Read the model definition and answer for the solid it produces. Units are mm, in the model's axes. A direction names the side the tool comes from. Round coordinates to 2 decimals unless told otherwise and drop trailing zeros. Loops run counter-clockwise (first coordinate to the right, second up) from the corner with the lowest first, then second, coordinate; pieces in that order, holes last. Notation, with made-up numbers: (28.25, 71.5) -> (32.25, 71.5) arc R17 cw to (32.25, 77.5) -> close; hole circle Ø9 at (53.5, 66.5). An arc over 180 degrees is marked (long way). Put each result on its own line as item: value.
from build123d import *

# Parameters (mm, degrees)
F0_W         = 20
F0_H         = 20
F0_R         = 8.25
F1_DEPTH     = 28.5
F0_R_2       = 4.75
F2_DEPTH     = 1.5
F3_W         = 9
F3_H         = 17.5
F3_R         = 1.6
F4_DEPTH     = 10
F5_W         = 9
F5_H         = 17.5
F6_DEPTH     = 10
F7_DEPTH     = 30.001
F8_R         = 5
F9_T1_DEPTH  = 22.5
F10_T1_DEPTH = 22.5
F11_R        = 1


# Not quite as in the source:
# - a fillet or chamfer that OpenCascade refuses, or shapes differently, is made with other operations: its cross-section is extruded or revolved along the edge and cut away or added


with BuildPart() as f1:
    # F0 (on Top) → F1 (new body)
    with BuildSketch(Plane.XY):
        Rectangle(F0_W, F0_H)
        Circle(F0_R, mode=Mode.SUBTRACT)
    extrude(amount=F1_DEPTH)

    # F0 (on Top) → F2 (join)
    with BuildSketch(Plane.XY):
        Circle(F0_R)
        Circle(F0_R_2, mode=Mode.SUBTRACT)
    extrude(amount=F2_DEPTH)

    # F3 (on face) → F4 (join)
    with BuildSketch(Plane(origin=(-10, 0, 0), x_dir=(0, -1, 0), z_dir=(-1, 0, 0))):
        with Locations((0, 8.75)):
            Rectangle(F3_W, F3_H)
        with Locations((0, 8.75)):
            Circle(F3_R, mode=Mode.SUBTRACT)
    extrude(amount=F4_DEPTH)

    # F5 (on face) → F6 (join)
    with BuildSketch(Plane.YZ.offset(10)):
        with Locations((0, 8.75)):
            Rectangle(F5_W, F5_H)
    extrude(amount=F6_DEPTH)

    # F3 (on face) → F7 (cut, through all)
    with BuildSketch(Plane(origin=(-10, 0, 0), x_dir=(0, -1, 0), z_dir=(-1, 0, 0))):
        with Locations((0, 8.75)):
            Circle(F3_R)
    extrude(amount=-F7_DEPTH, mode=Mode.SUBTRACT)

    # F8
    f8_edges = [f1.edges().sort_by_distance(p)[0] for p in [
        (-10, -10, 14.25),
        (10, -10, 14.25),
        (10, 10, 14.25),
        (-10, 10, 14.25),
    ]]
    fillet(f8_edges, radius=F8_R)

    # F9: fillet of radius 5 on 2 edges, made by hand

    # F9_s2 → F9_t1 (cut)
    with BuildSketch(Plane.YZ.offset(10)):
        with BuildLine():
            ThreePointArc((-4.5, 12.5), (-3.0355339059, 16.0355339059), (0.5, 17.5))
            Line((0.5, 17.5), (-4.5, 17.5))
            Line((-4.5, 17.5), (-4.5, 12.5))
        make_face()
        with BuildLine():
            ThreePointArc((-0.5, 17.5), (3.0355339059, 16.0355339059), (4.5, 12.5))
            Line((4.5, 12.5), (4.5, 17.5))
            Line((4.5, 17.5), (-0.5, 17.5))
        make_face()
    extrude(amount=F9_T1_DEPTH, mode=Mode.SUBTRACT)

    # F10: fillet of radius 5 on 2 edges, made by hand

    # F10_s2 → F10_t1 (cut)
    with BuildSketch(Plane.YZ.offset(-32.5)):
        with BuildLine():
            ThreePointArc((-4.5, 12.5), (-3.0355339059, 16.0355339059), (0.5, 17.5))
            Line((0.5, 17.5), (-4.5, 17.5))
            Line((-4.5, 17.5), (-4.5, 12.5))
        make_face()
        with BuildLine():
            ThreePointArc((4.5, 12.5), (3.0355339059, 16.0355339059), (-0.5, 17.5))
            Line((-0.5, 17.5), (4.5, 17.5))
            Line((4.5, 17.5), (4.5, 12.5))
        make_face()
    extrude(amount=F10_T1_DEPTH, mode=Mode.SUBTRACT)

    # F11
    f11_edges = [f1.edges().sort_by_distance(p)[0] for p in [
        (15, -4.5, 0),
        (15, 4.5, 0),
        (-15, 4.5, 0),
        (-15, -4.5, 0),
    ]]
    fillet(f11_edges, radius=F11_R)


solid = f1.part
Item 1: The part is cut by section D-D (z = 27). Determine the outline of the cut face in (x, y).
Derived:
outline: (-10, -5) arc R5 ccw to (-5, -10) -> (5, -10) arc R5 ccw to (10, -5) -> (10, 5) arc R5 ccw to (5, 10) -> (-5, 10) arc R5 ccw to (-10, 5) -> close; hole circle Ø16.5 at (0, 0)
Item 2: Find the intervals of material crossed by line 1 along Z through (x, y) = (13.75, 0); line 2 along Z through (x, y) = (-9.35, 0); line 3 along Y through (x, z) = (0, 16.5), in increasing order.
Derived:
line 1: z = 0 to 7.15, 10.35 to 17.47
line 2: z = 0 to 7.15, 10.35 to 28.5
line 3: y = -10 to -8.25, 8.25 to 10
Item 3: The part is cut by section B-B (x = 0). Determine the outline of the cut face in (y, z).
Derived:
outline: (-10, 0) -> (-4.75, 0) -> (-4.75, 1.5) -> (-8.25, 1.5) -> (-8.25, 28.5) -> (-10, 28.5) -> close; (4.75, 0) -> (10, 0) -> (10, 28.5) -> (8.25, 28.5) -> (8.25, 1.5) -> (4.75, 1.5) -> close
Item 4: The part is cut by section A-A (z = 8.75). Determine the outline of the cut face in (x, y).
Derived:
outline: (-20, -4.5) -> (-10, -4.5) -> (-10, -5) arc R5 ccw to (-5, -10) -> (5, -10) arc R5 ccw to (10, -5) -> (10, -4.5) -> (20, -4.5) -> (20, -1.6) -> (8.09, -1.6) arc R8.25 cw to (-8.09, -1.6) -> (-20, -1.6) -> close; (-20, 1.6) -> (-8.09, 1.6) arc R8.25 cw to (8.09, 1.6) -> (20, 1.6) -> (20, 4.5) -> (10, 4.5) -> (10, 5) arc R5 ccw to (5, 10) -> (-5, 10) arc R5 ccw to (-10, 5) -> (-10, 4.5) -> (-20, 4.5) -> close
Item 5: Flat-ended cylindrical pins translate along their axes: pin 1 Ø8 at (x, z) = (-12.5, 4.5) entering from -Y; pin 2 Ø3 at (y, z) = (0, 8.75) entering from -X; pin 3 Ø3 at (x, y) = (12, 2.5) entering from +Z; pin 4 Ø1 at (y, z) = (6, 15.5) entering from +X. Find the tip coordinate at first contact, or state that the pin passes through.
Derived:
pin 1: stops at y = -8.57
pin 2: passes through
pin 3: stops at z = 17.27
pin 4: stops at x = 9.97
Item 6: Which of the six approach directions +Z, -Z, +X, -X, +Y, -Y give full straight-line access (tool end or side, diameter ignored) to faces 5 (the flat face through (-15, -4.5, 7)), 6 (the cylindrical face through (-15.07, -3.24, 15.82)), 7 (the cylindrical face through (14.93, 3.173, 15.892)), 8 (the cylindrical face through (-15.07, -4.199, 0.285)), 9 (the cylindrical face through (-15.07, 4.199, 0.285))?
Derived:
face 5: +Z, -Z, -X, -Y
face 6: +Z, -X, -Y
face 7: +Z, +X, +Y
face 8: -Z, -X, -Y
face 9: -Z, -X, +Y
Item 7: The part is cut by section C-C (x = 14). Determine the outline of the cut face in (y, z), then the cut area to 3 significant figures.
Derived:
outline: (-4.5, 1) arc R1 ccw to (-3.5, 0) -> (3.5, 0) arc R1 ccw to (4.5, 1) -> (4.5, 12.5) arc R5 ccw to (0, 17.47) arc R5 ccw to (-4.5, 12.5) -> close; hole circle Ø3.2 at (0, 8.75)
area: 138 mm^2
Item 8: For a pull along Y with two mould halves and no side action, classify faces 1 (the cylindrical face through (15.07, -4.199, 0.285)), 2 (the cylindrical face through (7.87, 2.48, 14.81)), 3 (the cylindrical face through (15.07, 4.199, 0.285)), 4 (the flat face through (-9, 0, 28.5)) as pulls with the +Y half, pulls with the -Y half, needs draft (parallel to the pull), parting line crosses it, or undercut.
Derived:
face 1: pulls with the -Y half
face 2: undercut
face 3: pulls with the +Y half
face 4: needs draft
